Work out the finished part from the listing and answer in its coordinate system (mm). Face numbers are marked on the shaded views. A direction names the side the tool comes from. Coordinates: 2 decimals unless noted, no trailing zeros. Order: outer loops, then holes, each group sorted by start corner. A loop starts at its lowest first (then second) coordinate and runs counter-clockwise, first axis right, second up. Notation, with made-up numbers: M 66.25,9.25 L 86.25,9.25 A23 cw 86.25,20.25 Z; hole C -10,-27.5 d9. An arc over 180 degrees is marked long. Answer in a Markdown table with one row per item. Add a question column.
Item 1: The part is cut by section C-C (x = -44.45). Write down the section's boundary in (y, z) (3 decimals), then the cut area to 3 significant figures.
Item 2: The part is cut by section D-D (y = -7.75). Write down the section's boundary in (x, z), then the cut area to 3 significant figures.
Item 3: Consider line 1 (Y direction, x = -30.5, z = 16.5); line 2 (Z direction, x = -13, y = -7.75); line 3 (X direction, y = -8.25, z = 30). Determine where each line is inside the solid, lowest interval first. Write a range as from..to.
Item 4: The part is cut by section A-A (y = -16.75). Write down the section's boundary in (x, z) (3 decimals).
Item 5: The part is cut by section B-B (z = 3.81). Write down the section's boundary in (x, y) (3 decimals).
Item 6: Which of the six approach directions +Z, -Z, +X, -X, +Y, -Y give full straight-line access (tool end or side, diameter ignored) to the marked faces 1, 2 and 3?
Item 7: Flat-ended cylindrical pins translate along their axes: pin 1 Ø4 at (y, z) = (-7.5, 20.5) entering from +X; pin 2 Ø10 at (x, y) = (-14.5, -3.5) entering from +Z; pin 3 Ø19 at (x, z) = (-31.5, 26.5) entering from -Y. Find the tip coordinate at first contact, or state that the pin passes through.
Item 8: The mould has two halves that part along Z. Classify the marked faces 4, 5 and 6: released by +Z, released by -Z, zero draft, split by the parting line, or undercut.
from build123d import *

# Parameters (mm, degrees)
F1_DEPTH = 12.7
F2_R     = 3.175
F3_DEPTH = 6.35


with BuildPart() as f1:
    # F0 (on Front) → F1 (new body)
    with BuildSketch(Plane.XZ):
        Polygon((-50.8, 0), (0, 0), (0, 12.7), (-25.4, 12.7), (-25.4, 38.1), (-50.8, 38.1), align=None)
    extrude(amount=F1_DEPTH)

    # F2 (on face) → F3 (join)
    with BuildSketch(Plane.XZ.offset(12.7)):
        with Locations((-44.45, 3.81)):
            Circle(F2_R)
        with BuildLine():
            ThreePointArc((-28.575, 3.81), (-31.75, 6.985), (-34.925, 3.81))
            ThreePointArc((-34.925, 3.81), (-31.75, 0.635), (-28.575, 3.81))
        make_face()
    extrude(amount=F3_DEPTH)


solid = f1.part
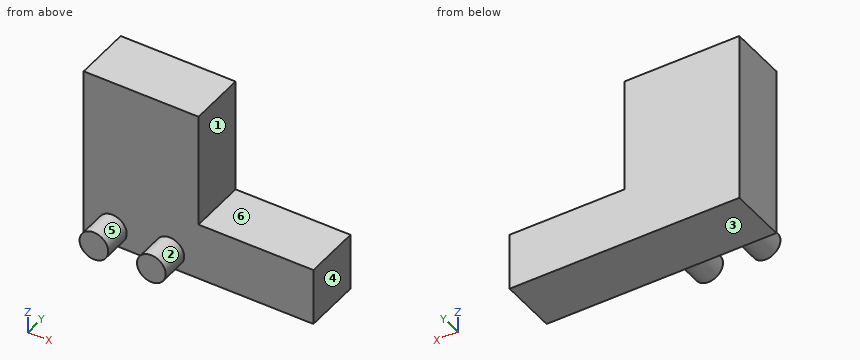
Reply:
| question | item | result |
|---|---|---|
| 1 | outline | M -19.05,0.635 L -12.7,0.635 L -12.7,0 L 0,0 L 0,38.1 L -12.7,38.1 L -12.7,6.985 L -19.05,6.985 Z |
| 1 | area | 524 mm2 |
| 2 | outline | M -50.8,0 L 0,0 L 0,12.7 L -25.4,12.7 L -25.4,38.1 L -50.8,38.1 Z |
| 2 | area | 1,290 mm2 |
| 3 | line 1 | y = -12.7..0 |
| 3 | line 2 | z = 0..12.7 |
| 3 | line 3 | x = -50.8..-25.4 |
| 4 | outline | C -44.45,3.81 d6.35; C -31.75,3.81 d6.35 |
| 5 | outline | M -50.8,-12.7 L -47.625,-12.7 L -47.625,-19.05 L -41.275,-19.05 L -41.275,-12.7 L -34.925,-12.7 L -34.925,-19.05 L -28.575,-19.05 L -28.575,-12.7 L 0,-12.7 L 0,0 L -50.8,0 Z |
| 6 | face 1 | +Z, +X, +Y, -Y |
| 6 | face 2 | -Y |
| 6 | face 3 | -Z, +X, -X, +Y, -Y |
| 7 | pin 1 | stops at x = -25.4 |
| 7 | pin 2 | stops at z = 12.7 |
| 7 | pin 3 | stops at y = -12.7 |
| 8 | face 4 | zero draft |
| 8 | face 5 | split by the parting line |
| 8 | face 6 | released by +Z |
